Geometry: final body of the model. Coordinates: model frame, mm. Face numbers are marked on the shaded views. A direction names the side the tool comes from. Round coordinates to 2 decimals unless told otherwise and drop trailing zeros. Loops run counter-clockwise (first coordinate to the right, second up) from the corner with the lowest first, then second, coordinate; pieces in that order, holes last. Notation, with made-up numbers: M 36,51 L 81,51 A18 ccw 81,58 Z; hole C 41.5,45.5 d8. An arc over 180 degrees is marked long. Write each question's results on one line, items separated by ' | '.
```python
from build123d import *

# Parameters (mm, degrees)
CROQUIS1_W              = 42
CROQUIS1_H              = 23
CROQUIS1_W_2            = 36
CROQUIS1_H_2            = 17
SALIENTE_EXTRUIR1_DEPTH = 70
REDONDEO1_R             = 3
REDONDEO2_R             = 1
CHAFL_N1_SIZE           = 0.5


with BuildPart() as part:
    # Croquis1 → Saliente-Extruir1 (new body)
    with BuildSketch(Plane(origin=(0, 0, 0), x_dir=(1, 0, 0), z_dir=(0, 1, 0))):
        Rectangle(CROQUIS1_W, CROQUIS1_H)
        Rectangle(CROQUIS1_W_2, CROQUIS1_H_2, mode=Mode.SUBTRACT)
    extrude(amount=SALIENTE_EXTRUIR1_DEPTH)

    # Redondeo1
    redondeo1_edges = [part.edges().sort_by_distance(p)[0] for p in [
        (-21, 35, -11.5),
        (21, 35, -11.5),
        (21, 35, 11.5),
        (-21, 35, 11.5),
    ]]
    fillet(redondeo1_edges, radius=REDONDEO1_R)

    # Redondeo2
    redondeo2_edges = [part.edges().sort_by_distance(p)[0] for p in [
        (18, 35, 8.5),
        (18, 35, -8.5),
        (-18, 35, -8.5),
        (-18, 35, 8.5),
    ]]
    fillet(redondeo2_edges, radius=REDONDEO2_R)

    # Chaflán1
    chafl_n1_edges = [part.edges().sort_by_distance(p)[0] for p in [
        (-21, 0, 0),
        (-21, 70, 0),
        (0, 0, -11.5),
        (21, 0, 0),
        (0, 0, 11.5),
        (-20.121320344, 0, 10.621320344),
        (20.121320344, 0, 10.621320344),
        (20.121320344, 0, -10.621320344),
        (-20.121320344, 0, -10.621320344),
        (0, 70, -11.5),
        (0, 70, 11.5),
        (21, 70, 0),
        (-20.121320344, 70, 10.621320344),
        (20.121320344, 70, 10.621320344),
        (20.121320344, 70, -10.621320344),
        (-20.121320344, 70, -10.621320344),
        (0, 0, 8.5),
        (0, 70, 8.5),
        (18, 0, 0),
        (18, 70, 0),
        (0, 0, -8.5),
        (0, 70, -8.5),
        (-18, 0, 0),
        (-18, 70, 0),
        (17.707106781, 0, 8.207106781),
        (17.707106781, 70, 8.207106781),
        (17.707106781, 0, -8.207106781),
        (17.707106781, 70, -8.207106781),
        (-17.707106781, 0, -8.207106781),
        (-17.707106781, 70, -8.207106781),
        (-17.707106781, 0, 8.207106781),
        (-17.707106781, 70, 8.207106781),
    ]]
    chamfer(chafl_n1_edges, length=CHAFL_N1_SIZE)


solid = part.part
```
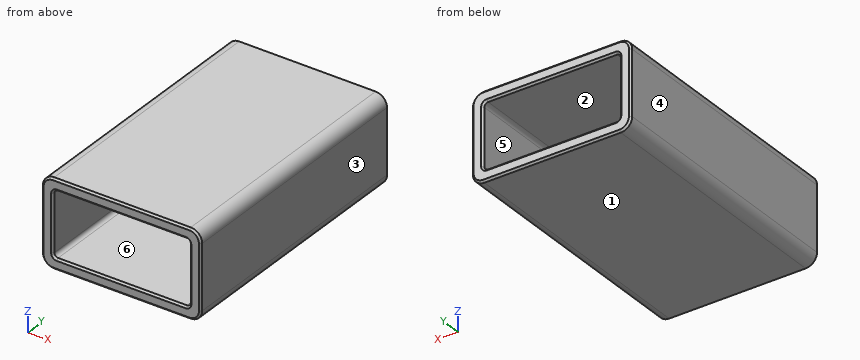
1. Draft query along X for the marked faces 3, 4, 5 and 6. Return one class per face: pulls with the +X half, pulls with the -X half, needs draft (parallel to the pull), parting line crosses it, or undercut.
Answer key:
face 3: pulls with the +X half | face 4: pulls with the -X half | face 5: undercut | face 6: undercut
2. Section C-C (y = 30). Output: boundary loops of the cut face in (x, z).
Answer key:
outline: M -21,-8.5 A3 ccw -18,-11.5 L 18,-11.5 A3 ccw 21,-8.5 L 21,8.5 A3 ccw 18,11.5 L -18,11.5 A3 ccw -21,8.5 Z; hole M -18,-7.5 A1 ccw -17,-8.5 L 17,-8.5 A1 ccw 18,-7.5 L 18,7.5 A1 ccw 17,8.5 L -17,8.5 A1 ccw -18,7.5 Z
3. Ray query, probe 1 along X at (y, z) = (19.5, -2.75); probe 2 along Z at (x, y) = (-5.5, 22); probe 3 along X at (y, z) = (63, 8). Return the intervals inside material, ascending.
Answer key:
probe 1: x = -21 to -18, 18 to 21 | probe 2: z = -11.5 to -8.5, 8.5 to 11.5 | probe 3: x = -21 to -17.87, 17.87 to 21
4. Access query for the marked faces 1 and 2. Directions: +Z, -Z, +X, -X, +Y, -Y. A direction counts if a zero-diameter tool reaches every point of the face in a straight line with its end or side. Return the directions, or none.
Answer key:
face 1: -Z, +X, -X, +Y, -Y | face 2: +Y, -Y
5. Section A-A (x = -11). Output: boundary loops of the cut face in (y, z).
Answer key:
outline: M 0,-11 L 0.5,-11.5 L 69.5,-11.5 L 70,-11 L 70,-9 L 69.5,-8.5 L 0.5,-8.5 L 0,-9 Z; M 0,9 L 0.5,8.5 L 69.5,8.5 L 70,9 L 70,11 L 69.5,11.5 L 0.5,11.5 L 0,11 Z
6. Section B-B (z = 5.75). Output: boundary loops of the cut face in (x, y).
Answer key:
outline: M -21,0.5 L -20.5,0 L -18.5,0 L -18,0.5 L -18,69.5 L -18.5,70 L -20.5,70 L -21,69.5 Z; M 18,0.5 L 18.5,0 L 20.5,0 L 21,0.5 L 21,69.5 L 20.5,70 L 18.5,70 L 18,69.5 Z
